Answer from the drawing. Dimensions are ordinates in mm from the lowest x, y and z of the part. A direction names the side the tool comes from. Coordinates: 2 decimals unless noted, no trailing zeros. Order: outer loops, then holes, each group sorted by start corner. A loop starts at its lowest first (then second) coordinate and runs counter-clockwise, first axis right, second up. Notation, with made-up numbers: (21.25, 40) -> (37.25, 40) arc R26 cw to (37.25, 75) -> close; hole circle Ø7 at (35.25, 23.5). An arc over 180 degrees is marked (long way). Answer in a Markdown table with one row per item.
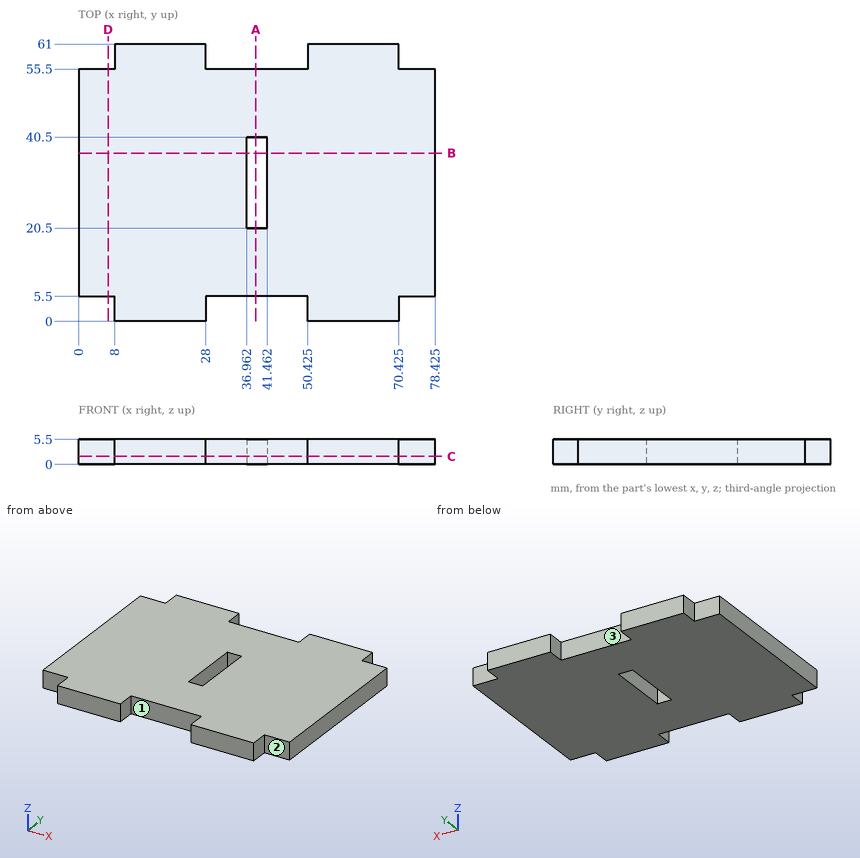
Q1. The part is cut by section A-A (x = 39). Write down the section's boundary in (y, z).
Outcome:
| item | result |
|---|---|
| outline | (5.5, 0) -> (20.5, 0) -> (20.5, 5.5) -> (5.5, 5.5) -> close; (40.5, 0) -> (55.5, 0) -> (55.5, 5.5) -> (40.5, 5.5) -> close |
Q2. The part is cut by section B-B (y = 37). Write down the section's boundary in (x, z) (1 decimal).
Outcome:
| item | result |
|---|---|
| outline | (0, 0) -> (37, 0) -> (37, 5.5) -> (0, 5.5) -> close; (41.5, 0) -> (78.4, 0) -> (78.4, 5.5) -> (41.5, 5.5) -> close |
Q3. For the marked faces 1, 2 and 3, determine the directions among +Z, -Z, +X, -X, +Y, -Y from which every point of the face is accessible in a straight line to the end or side of a thin tool.
Outcome:
| item | result |
|---|---|
| face 1 | +Z, -Z, -Y |
| face 2 | +Z, -Z, +X, -Y |
| face 3 | +Z, -Z, +Y |
Q4. Given pin 1 (1.5 mm diameter, centred on x = 36.5, z = 4, fed in from +Y); pin 2 (3 mm diameter, centred on x = 40.5, z = 3.5, fed in from -Y); pin 3 (3 mm diameter, centred on y = 58, z = 2.5, fed in from -X), each flat-ended and moving along its own axis, determine where each tip first touches the part or whether it passes through.
Outcome:
| item | result |
|---|---|
| pin 1 | y = 55.5 |
| pin 2 | y = 5.5 |
| pin 3 | x = 8 |
Q5. Consider line 1 (X direction, y = 28, z = 0.65) (1 decimal); line 2 (X direction, y = 57.5, z = 5.3) (1 decimal); line 3 (Y direction, x = 35, z = 2.35). Determine where each line is inside the solid, lowest interval first.
Outcome:
| item | result |
|---|---|
| line 1 | 0 to 37, 41.5 to 78.4 |
| line 2 | 8 to 28, 50.4 to 70.4 |
| line 3 | 5.5 to 55.5 |
Q6. The part is cut by section C-C (z = 1.75). Write down the section's boundary in (x, y) (1 decimal), then the cut area to 3 significant figures.
Outcome:
| item | result |
|---|---|
| outline | (0, 5.5) -> (8, 5.5) -> (8, 0) -> (28, 0) -> (28, 5.5) -> (50.4, 5.5) -> (50.4, 0) -> (70.4, 0) -> (70.4, 5.5) -> (78.4, 5.5) -> (78.4, 55.5) -> (70.4, 55.5) -> (70.4, 61) -> (50.4, 61) -> (50.4, 55.5) -> (28, 55.5) -> (28, 61) -> (8, 61) -> (8, 55.5) -> (0, 55.5) -> close; hole (37, 20.5) -> (41.5, 20.5) -> (41.5, 40.5) -> (37, 40.5) -> close |
| area | 4,270 mm² |
Q7. The part is cut by section D-D (x = 6.5). Write down the section's boundary in (y, z).
Outcome:
| item | result |
|---|---|
| outline | (5.5, 0) -> (55.5, 0) -> (55.5, 5.5) -> (5.5, 5.5) -> close |
